Design review of the part built by this model. Coordinates are the model's own, in mm. Face numbers are marked on the shaded views. Round coordinates to 2 decimals unless told otherwise and drop trailing zeros. Order: outer loops, then holes, each group sorted by start corner. A loop starts at its lowest first (then second) coordinate and runs counter-clockwise, first axis right, second up. Notation, with made-up numbers: (44, -39) - (67, -39) arc R27 ccw to (67, -12) - close; hole circle Ø9 at (13, 13.25). An arc over 180 degrees is marked (long way). Write item = value, one per line.
from build123d import *

# Parameters (mm, degrees)
F0_W        = 1462
F0_H        = 1610
F1_DEPTH    = 77
F3_W        = 1750
F3_H        = 1524
F4_DEPTH    = 77
F1_FACE_W   = 1462
F1_FACE_H   = 1610
F4_FACE_W   = 1750
F4_FACE_H   = 1524
F6_T        = 3
F6_T3_DEPTH = 1756
F6_T5_DEPTH = 1616


# Not quite as in the source:
# - a shell that OpenCascade refuses in one call is made with other operations: the cavity is built on its own and cut out


with BuildPart() as f1:
    # F0 (on Front) → F1 (new body)
    with BuildSketch(Plane.XZ):
        with Locations((0, 805)):
            Rectangle(F0_W, F0_H)
    extrude(amount=-F1_DEPTH)



with BuildPart() as f4:
    # F3 (on offset) → F4 (new body)
    with BuildSketch(Plane(origin=(0, 317, 0), x_dir=(-1, 0, 0), z_dir=(0, 1, 0))):
        with Locations((0, 762)):
            Rectangle(F3_W, F3_H)
    extrude(amount=F4_DEPTH)


with BuildPart() as f1_1:
    add(f1.part)

    add(f4.part)  # F5 merges F4
    # F1_face (on face) → F5 section 0
    with BuildSketch(Plane(origin=(0, 77, 805), x_dir=(1, 0, 0), z_dir=(0, 1, 0))):
        Rectangle(F1_FACE_W, F1_FACE_H)
    # F4_face (on face) → F5 section 1
    with BuildSketch(Plane(origin=(0, 317, 762), x_dir=(-1, 0, 0), z_dir=(0, -1, 0))):
        Rectangle(F4_FACE_W, F4_FACE_H)
    loft()

    # F6: shell of thickness 3, made by hand


with BuildPart() as f6_core1:
    # F6_t2: copy of F1
    add(f1_1.part)

    # the walls: a layer under each face that stays
    f6_faces = [f6_core1.faces().sort_by_distance(p)[0] for p in [
        (0, 197, 0),
        (875, 355.5, 762),
        (-875, 355.5, 762),
        (0, 355.5, 1524),
        (803, 197, 783.5),
        (-803, 197, 783.5),
        (-731, 38.5, 805),
        (731, 38.5, 805),
        (0, 197, 1567),
        (0, 38.5, 1610),
    ]]
    thicken(f6_faces, amount=-F6_T, mode=Mode.SUBTRACT)

    # F6_s4 → F6_t3 (cut)
    with BuildSketch(Plane.YZ.offset(-878)):
        Polygon((317.010119904, 1524.0582415924), (317, 1521), (316.4787279914, 1521), (315.988009604, 1521.1758407555), align=None)
    extrude(amount=F6_T3_DEPTH, mode=Mode.SUBTRACT)

    # F6_s6 → F6_t5 (cut)
    with BuildSketch(Plane.XY.offset(-3)):
        Polygon((731.0557247878, 76.9845651273), (728.4275212229, 78.5434872663), (728, 77.8309518948), (728, 77), align=None)
        Polygon((-731.0557247878, 76.9845651273), (-728.4275212229, 78.5434872663), (-728, 77.8309518948), (-728, 77), align=None)
    extrude(amount=F6_T5_DEPTH, mode=Mode.SUBTRACT)


with BuildPart() as f1_2:
    add(f1_1.part)

    # what is left inside the walls is the cavity
    f6_cavity = [f6_core1.part.solids().sort_by_distance(p)[0] for p in [
        (0, 393.97, 509),
    ]]
    add(f6_cavity, mode=Mode.SUBTRACT)


solid = f1_2.part
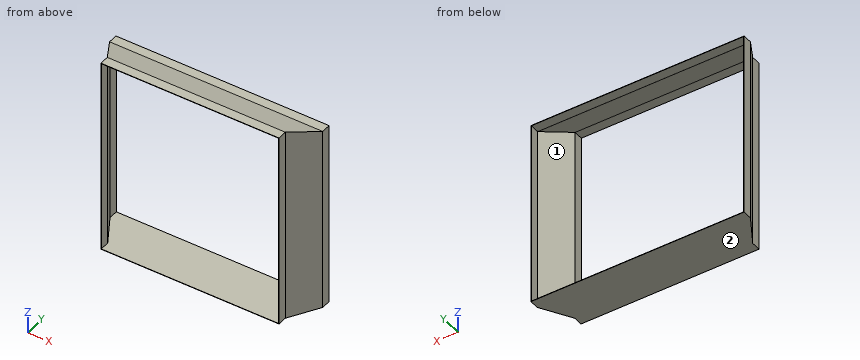
Item 1: Take a section at A-A, the plane y = 50. State the section outline as (x, z) points.
Data:
outline = (-731, 0) - (731, 0) - (731, 1610) - (-731, 1610) - close; hole (-728, 3) - (728, 3) - (728, 1607) - (-728, 1607) - close
Item 2: For line 1 along X through (y, z) = (68, 671); line 2 along Z through (x, y) = (-22, 65.5); line 3 along X through (y, z) = (356, 663), list the stretches that pass through material, from the lowest coordinate up. Write a range as [from, to].
Data:
line_1 = [-731, -728], [728, 731]
line_2 = [0, 3], [1607, 1610]
line_3 = [-875, -872], [872, 875]
Item 3: Take a section at B-B, the plane y = 367. State the section outline as (x, z) points, and give its area (3 significant figures).
Data:
outline = (-875, 0) - (875, 0) - (875, 1524) - (-875, 1524) - close; hole (-872, 3) - (872, 3) - (872, 1521) - (-872, 1521) - close
area = 19,600 mm2
Item 4: Insertion check: P1, Ø5, axis at x = -658, y = 104, coming from the +Z side; P2, Ø8, axis at y = 211, z = 904, coming from the -X side; P3, Ø4, axis at y = 49, z = 1158.5, coming from the +X side. Each pin has a flat end and moves straight along its axis. Give the tip position at first contact, or say it passes through.
Data:
P1 = 1601.22
P2 = -813.8
P3 = 731
Item 5: The part is to be moulded in two halves that separate along X. For the marked faces 1 and 2, say which applies: +X half, -X half, draft (parallel to the pull), parting line (faces both ways), or undercut.
Data:
face_1 = undercut
face_2 = draft
